```python
from build123d import *

# Parameters (mm, degrees)
F0_W     = 60
F0_H     = 60
F1_DEPTH = 30
F1_TAPER = 45
F2_W     = 80
F2_H     = 80
F2_W_2   = 60
F2_H_2   = 60
F3_DEPTH = 6.35


with BuildPart() as f1:
    # F0 (on Top) → F1 (new body)
    with BuildSketch(Plane.XY):
        Rectangle(F0_W, F0_H)
    extrude(amount=F1_DEPTH, taper=F1_TAPER)

    # F2 (on face) → F3 (join)
    with BuildSketch(Plane(origin=(0, 0, 0), x_dir=(1, 0, 0), z_dir=(0, 0, -1))):
        Rectangle(F2_W, F2_H)
        Rectangle(F2_W_2, F2_H_2, mode=Mode.SUBTRACT)
        Rectangle(F2_W_2, F2_H_2)
    extrude(amount=F3_DEPTH)


solid = f1.part
```
Input: part model. Units: mm. Frame: model coordinates. A direction names the side the tool comes from. Coordinates: 2 decimals unless noted, no trailing zeros. Loops run counter-clockwise (first coordinate to the right, second up) from the corner with the lowest first, then second, coordinate; pieces in that order, holes last. Notation, with made-up numbers: M 21,-12.5 L 28,-12.5 A13 ccw 28,-4.5 Z; hole C 31,-6.5 d6. An arc over 180 degrees is marked long. Answer in a Markdown table with one row per item.
1. First-contact query: pin 1 (12 mm diameter, centred on y = 17.5, z = 13.5, fed in from -X); pin 2 (1 mm diameter, centred on y = 9.5, z = 4.5, fed in from -X); pin 3 (5 mm diameter, centred on x = -7, z = 6, fed in from +Y). Flat tips, straight axial feed; report the tip coordinate or a pass-through.
Response:
| item | result |
|---|---|
| pin 1 | stops at x = -22.5 |
| pin 2 | stops at x = -26 |
| pin 3 | stops at y = 26.5 |
2. Material intervals for line 1 (Z direction, x = 30.5, y = -4); line 2 (Y direction, x = -1, z = 26); line 3 (Y direction, x = 3.5, z = 12.5), sorted ascending.
Response:
| item | result |
|---|---|
| line 1 | z = -6.35 to 0 |
| line 2 | y = -4 to 4 |
| line 3 | y = -17.5 to 17.5 |
3. Section D-D, the plane x = -32.5. Output: boundary loops of the cut face in (y, z), then the cut area to 3 significant figures.
Response:
| item | result |
|---|---|
| outline | M -40,-6.35 L 40,-6.35 L 40,0 L -40,0 Z |
| area | 508 mm2 |
4. Section B-B, the plane x = 13.5. Output: boundary loops of the cut face in (y, z).
Response:
| item | result |
|---|---|
| outline | M -40,-6.35 L 40,-6.35 L 40,0 L 30,0 L 13.5,16.5 L -13.5,16.5 L -30,0 L -40,0 Z |
5. Reachability of faces 1 (the flat face through (-36, -1, 0)), 2 (the flat face through (19, 0, 11)) from +Z, -Z, +X, -X, +Y, -Y: full face, straight path, thin tool, end or side. Return the list, or none.
Response:
| item | result |
|---|---|
| face 1 | +Z |
| face 2 | +Z, +X, +Y, -Y |
6. Section C-C, the plane z = 25. Output: boundary loops of the cut face in (x, y).
Response:
| item | result |
|---|---|
| outline | M -5,-5 L 5,-5 L 5,5 L -5,5 Z |
7. Section A-A, the plane y = -29. Output: boundary loops of the cut face in (x, z), then the cut area to 3 significant figures.
Response:
| item | result |
|---|---|
| outline | M -40,-6.35 L 40,-6.35 L 40,0 L 30,0 L 29,1 L -29,1 L -30,0 L -40,0 Z |
| area | 567 mm2 |
